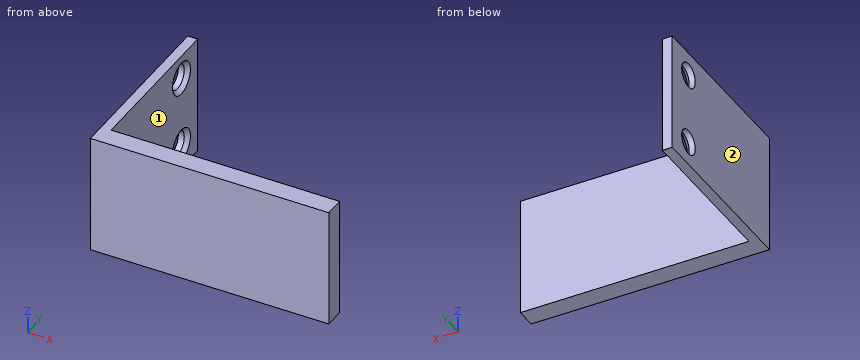
from build123d import *

# Parameters (mm, degrees)
SKETCH_1_W                    = 12
SKETCH_1_H                    = 6
EXTRUDE_1_DEPTH               = 1
SKETCH_2_W                    = 0.5
SKETCH_2_H                    = 6
EXTRUDE_2_DEPTH               = 8
HOLE_WIZARD_M1_6_1_AT_2_COUNT = 2
HOLE_WIZARD_M1_6_1_AT_2_PITCH = 3.6


with BuildPart() as part:
    # 草图1 → 凸台-拉伸1 (new body)
    with BuildSketch(Plane(origin=(0, 0, 0), x_dir=(1, 0, 0), z_dir=(0, 1, 0))):
        Rectangle(SKETCH_1_W, SKETCH_1_H)
    extrude(amount=EXTRUDE_1_DEPTH)

    # 草图2 → 凸台-拉伸2 (add)
    with BuildSketch(Plane(origin=(0, 1, 0), x_dir=(1, 0, 0), z_dir=(0, 1, 0))):
        with Locations((-5.75, 0)):
            Rectangle(SKETCH_2_W, SKETCH_2_H)
    extrude(amount=EXTRUDE_2_DEPTH)

    # 草图5 → M1.6 螺纹孔1 (revolve, cut)
    with BuildSketch(Plane(origin=(-5.5, 7.5, -1.8), x_dir=(0, 0, -1), z_dir=(0, 1, 0))):
        Polygon((0, 0), (0, 0.5), (0.625, 0.5), (0.625, 0.2), (0.825, 0), align=None)
    hole_wizard_m1_6_1 = revolve(axis=Axis((0.85, 7.5, -1.8), (-1, 0, 0)), mode=Mode.SUBTRACT)

    # M1.6 螺纹孔1 at 2: M1.6 螺纹孔1 ×2
    with Locations(*[(0, 0, i * HOLE_WIZARD_M1_6_1_AT_2_PITCH) for i in range(1, HOLE_WIZARD_M1_6_1_AT_2_COUNT)]):
        add(hole_wizard_m1_6_1, mode=Mode.SUBTRACT)


solid = part.part
Here's how the part is built. I have some questions about the finished solid (model axes, mm). Face numbers are marked on the shaded views. A direction names the side the tool comes from. Round coordinates to 2 decimals unless told otherwise and drop trailing zeros. Write each loop counter-clockwise with the first axis right and the second up, starting at its lowest first coordinate (ties: lowest second). Pieces come first, ordered by that corner, then holes.
1. For the marked faces 1 and 2, which set-ups out of +Z, -Z, +X, -X, +Y, -Y let a thin tool reach every point of the face, with its end or its side?
2. Suppose I cut it at A-A (y = 7.5). List the corners of the cut face in (x, z) for me (3 decimals), and give its area (3 significant figures).
3. Suppose I cut it at D-D (x = -3.25). List the corners of the cut face in (y, z) for me, and give its area (3 significant figures).
4. Suppose I cut it at C-C (z = -0.7). List the corners of the cut face in (x, y) for me.
5. Will these pins go through, and if not, where does the flat tip stop? pin 1 Ø2 at (x, z) = (-4, 1.5) entering from +Y; pin 2 Ø0.7 at (y, z) = (7.5, 1.8) entering from +X.
6. Suppose I cut it at B-B (z = 1.8). List the corners of the cut face in (x, y) for me (3 decimals), and give its area (3 significant figures).
7. I need wall thicknesses on L1, parallel to Z at x = -5.85, y = 7.5 (3 decimals); L2, parallel to Y at x = -5.85, z = -1.8 (3 decimals); L3, parallel to X at y = 6.75, z = 0.1. Which ranges of each line are inside material? Lowest first, please.
Answer sheet:
1. face 1: +Z, -Z, +X, +Y
1. face 2: +Z, -Z, -X, +Y, -Y
2. outline: (-6, -3) - (-5.5, -3) - (-5.5, -2.625) - (-5.7, -2.425) - (-6, -2.425) - close; (-6, -1.175) - (-5.7, -1.175) - (-5.5, -0.975) - (-5.5, 0.975) - (-5.7, 1.175) - (-6, 1.175) - close; (-6, 2.425) - (-5.7, 2.425) - (-5.5, 2.625) - (-5.5, 3) - (-6, 3) - close
2. area: 1.67 mm2
3. outline: (0, -3) - (1, -3) - (1, 3) - (0, 3) - close
3. area: 6.00 mm2
4. outline: (-6, 0) - (6, 0) - (6, 1) - (-5.5, 1) - (-5.5, 9) - (-6, 9) - close
5. pin 1: stops at y = 1
5. pin 2: passes through
6. outline: (-6, 0) - (6, 0) - (6, 1) - (-5.5, 1) - (-5.5, 6.675) - (-5.7, 6.875) - (-6, 6.875) - close; (-6, 8.125) - (-5.7, 8.125) - (-5.5, 8.325) - (-5.5, 9) - (-6, 9) - close
6. area: 15.3 mm2
7. L1: z = -3 to -2.425, -1.175 to 1.175, 2.425 to 3
7. L2: y = 0 to 6.875, 8.125 to 9
7. L3: x = -6 to -5.5
